```python
from build123d import *

# Parameters (mm, degrees)
HOLE_WIZARD_M51_D     = 4.2
HOLE_WIZARD_M51_DEPTH = 10


with BuildPart() as part:
    # Эскиз2 → Повернуть-Тонкостенный3 (revolve)
    with BuildSketch(Plane(origin=(0, 0, 0), x_dir=(0, 0, -1), z_dir=(1, 0, 0)), mode=Mode.PRIVATE) as revolve_3_sk:
        Polygon((-753, 35), (-450, 5), (-399, 5), (0, 5), (0, 7), (-399, 7), (-449.901231564, 7), (-752.80294371, 36.990268529), align=None)
    revolve(revolve_3_sk.sketch.rotate(Axis((0, 0, 1181.729856139), (0, 0, -1)), 90), axis=Axis((0, 0, 1181.729856139), (0, 0, -1)))

    # Эскиз8 → Повернуть1 (revolve)
    with BuildSketch(Plane(origin=(0, 0, 0), x_dir=(0, 0, -1), z_dir=(1, 0, 0)), mode=Mode.PRIVATE) as revolve_1_sk:
        Polygon((0, 5), (0, 35), (10, 35), (10, 15), (10, 5), align=None)
    revolve(revolve_1_sk.sketch.rotate(Axis((0, 0, 1181.729856139), (0, 0, -1)), 90), axis=Axis((0, 0, 1181.729856139), (0, 0, -1)))

    # Эскиз10 → Повернуть-Тонкостенный6 (revolve)
    with BuildSketch(Plane(origin=(0, 0, 0), x_dir=(0, 0, -1), z_dir=(1, 0, 0)), mode=Mode.PRIVATE) as revolve_6_sk:
        Polygon((0, 20), (-550, 20), (-554.567434607, 17.3629904), (-553.567434607, 15.630939593), (-549.464101615, 18), (0, 18), align=None)
    revolve(revolve_6_sk.sketch.rotate(Axis((0, 0, -54.408578324), (0, 0, 1)), 90), axis=Axis((0, 0, -54.408578324), (0, 0, 1)))

    # Отверстие обработанное метчиком M51
    with Locations(Plane.XY):
        with Locations((-23.815698604, 13.75), (0, 27.5), (23.815698604, 13.75), (23.815698604, -13.75), (-23.815698604, -13.75), (0, -27.5)):
            Hole(HOLE_WIZARD_M51_D / 2, depth=HOLE_WIZARD_M51_DEPTH)


solid = part.part
```
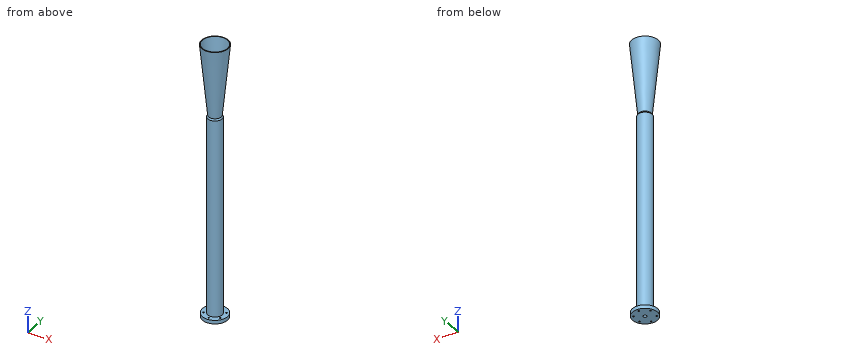
Part model, mm, in its own coordinate system. Round coordinates to 2 decimals unless told otherwise and drop trailing zeros. Write each loop counter-clockwise with the first axis right and the second up, starting at its lowest first coordinate (ties: lowest second). Pieces come first, ordered by that corner, then holes. Notation, with made-up numbers: (16.5, -13) -> (70.5, -13) arc R9 cw to (70.5, 2) -> close; hole circle Ø3 at (-8.5, 11). An arc over 180 degrees is marked (long way). Return JSON: item names as keys, results as strings. Group by question number.
Q1. Saw through at B-B on z = 639.5. Write the cut outline in (x, y), plus the area to 3 significant figures.
Q2. Probe L1, parallel to Y at x = 0, z = 332; L2, parallel to Y at x = 0, z = -4.5; L3, parallel to X at y = 2.5, z = 255. List the from-to ranges inside material, lowest first. Write a range as [from, to].
Q3. Pin check, flat tips, straight feed: pin 1 (4 mm diameter, centred on x = 10.5, z = 345, fed in from -Y); pin 2 (4 mm diameter, centred on y = 15.5, z = 150.5, fed in from +X); pin 3 (4 mm diameter, centred on x = -4.5, z = 259, fed in from +Y). Stop position of each tip, or through.
Q4. Saw through at A-A on z = 170. Write the cut outline in (x, y).
Q5. Saw through at C-C on z = 463. Write the cut outline in (x, y).
Answer:
{
 "1": {"outline": "circle Ø51.54 at (0, 0); hole circle Ø47.52 at (0, 0)", "area": "313 mm2"},
 "2": {"L1": "[-20, -18], [-7, -5], [5, 7], [18, 20]", "L2": "[-35, -29.6], [-25.4, -5], [5, 25.4], [29.6, 35]", "L3": "[-19.84, -17.83], [-6.54, -4.33], [4.33, 6.54], [17.83, 19.84]"},
 "3": {"pin 1": "y = -18.1", "pin 2": "x = 14.76", "pin 3": "y = 19.84"},
 "4": {"outline": "circle Ø40 at (0, 0); circle Ø14 at (0, 0); hole circle Ø36 at (0, 0); hole circle Ø10 at (0, 0)"},
 "5": {"outline": "circle Ø40 at (0, 0); circle Ø16.59 at (0, 0); hole circle Ø36 at (0, 0); hole circle Ø12.57 at (0, 0)"}
}
